Work out the finished part from the listing and answer in its coordinate system (mm). Face numbers are marked on the shaded views. A direction names the side the tool comes from. Coordinates: 2 decimals unless noted, no trailing zeros. Order: outer loops, then holes, each group sorted by start corner. A loop starts at its lowest first (then second) coordinate and runs counter-clockwise, first axis right, second up. Notation, with made-up numbers: M -27,51 L -11,51 A25 cw -11,84 Z; hole C 60.25,-28 d4. An arc over 180 degrees is marked long. Use a Markdown table: item, result.
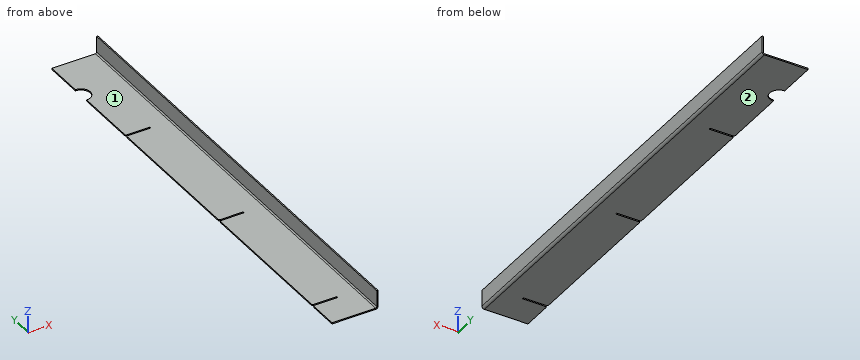
Autodesk Inventor part; units mm, degrees
ref_plane "YZ Plane" through (0, 0, 0) normal (1, 0, 0) x (0, 1, 0)
ref_plane "XZ Plane" through (0, 0, 0) normal (0, 1, 0) x (-1, 0, 0)
ref_plane "XY Plane" through (0, 0, 0) normal (0, 0, 1) x (1, 0, 0)
sketch "Sketch1" plane through (0, 0, 0) normal (0, 0, 1) x (1, 0, 0)
  line L0 (0, 0) -> (-144.8838, 0)
  line L1 (-144.8838, 0) -> (-144.8838, -1490)
  line L2 (-144.8838, -1490) -> (0, -1490)
  line L3 (0, -1490) -> (0, 0)
  line L4 (-144.8838, -1390) -> (-66, -1390)
  line L5 (-66, -1390) -> (-66, -1385)
  line L6 (-66, -1385) -> (-144.8838, -1385)
  line L7 (-144.8838, -1385) -> (-144.8838, -1390)
  line L8 (-144.8838, -893.3333) -> (-66, -893.3333)
  line L9 (-66, -893.3333) -> (-66, -888.3333)
  line L10 (-66, -888.3333) -> (-144.8838, -888.3333)
  line L11 (-144.8838, -888.3333) -> (-144.8838, -893.3333)
  line L12 (-144.8838, -396.6667) -> (-66, -396.6667)
  line L13 (-66, -396.6667) -> (-66, -391.6667)
  line L14 (-66, -391.6667) -> (-144.8838, -391.6667)
  line L15 (-144.8838, -391.6667) -> (-144.8838, -396.6667)
  circle A0 centre (-144.8838, -155) radius 30
  point P0 (-144.8838, -391.6667)
  point P1 (-144.8838, -1385)
  point P2 (-144.8838, -125)
  point P3 (-144.8838, -185)
  dimension "d0" = 1490
  dimension "d1" = 144.8838
  dimension "d2" = 5
  dimension "d4" = 100
  dimension "d7" = 496.6667
  dimension "d23" = 66
  dimension "d28" = 60
  dimension "d29" = 1335
extrude "Plate1" add sketch "Sketch1" along normal blind 4 contours L3 L2 L1 L4 L5 L6 L8 L9 L10 L12 L13 L14 A0 L0
sketch "Sketch2" plane through (4, 0, 0) normal (-1, 0, 0) x (0, -1, 0)
  line L0 (1490, 0) -> (0, 0)
  line L1 (0, 0) -> (0, 60)
  line L2 (0, 60) -> (1490, 60)
  line L3 (1490, 60) -> (1490, 0)
edge flange "Flange1" height 60 angle 90 thickness 4 bend radius 4 thickness toward (-1, 0, 0) relief tear relief width 4 relief depth 2 edges at (0, -745, 4) wall of the first edge with corners at (4, -1490, 0) (4, 0, 0) (4, 0, 60) (4, -1490, 60)
bend "Bend1"
corner "Corner1"
chamfer "Corner Chamfer1" distance 3 angle 45 6 edges at (-144.8838, -1390, 2) (-144.8838, -1385, 2) (-144.8838, -893.3333, 2) (-144.8838, -888.3333, 2) (-144.8838, -391.6667, 2) (-144.8838, -396.6667, 2)
equation "\"d0\" = Стрингер_длина"
equation "\"d1\" = стрингер_глубина_5"
equation "\"d2\" = паз_под_стрингер_толщина"
equation "\"d7\" = 0.333333 * Стрингер_длина"
equation "\"d23\" = паз_под_стрингер_глубина - Thickness"
equation "\"d28\" = 2 * радиус_выреза_под_сварку"
equation "\"d12\" = Thickness"
equation "\"d13\" = BendReliefWidth"
equation "\"d14\" = BendReliefDepth"
equation "\"d15\" = MinimumRemnant"
equation "\"d16\" = TransitionRadius"
equation "\"d17\" = ребро_усилителей"
equation "\"d19\" = BendRadius"
equation "\"d20\" = CornerReliefSize"
equation "\"d21\" = GapSize"
equation "\"d22\" = JacobiRadiusSize"
equation "\"BendRadius\" = Thickness"
equation "\"BendReliefWidth\" = Thickness"
equation "\"BendReliefDepth\" = 0.5 * Thickness"
equation "\"CornerReliefSize\" = 4 * Thickness"
equation "\"MinimumRemnant\" = 2 * Thickness"
equation "\"TransitionRadius\" = BendRadius"
equation "\"JacobiRadiusSize\" = BendRadius"
equation "\"GapSize\" = Thickness"
properties part number "GBK 0203 stringer 5" material "Steel"
1. Section C-C on x = -24.5 is taken. Determine the outline of the cut face in (y, z), then the cut area to 3 significant figures.
Answers below:
| item | result |
|---|---|
| outline | M -1490,0 L 0,0 L 0,4 L -1490,4 Z |
| area | 5,960 mm² |
2. Section D-D on z = 37.5 is taken. Determine the outline of the cut face in (x, y), then the cut area to 3 significant figures.
Answers below:
| item | result |
|---|---|
| outline | M 0,-1490 L 4,-1490 L 4,0 L 0,0 Z |
| area | 5,960 mm² |
3. Section A-A on x = -93 is taken. Determine the outline of the cut face in (y, z).
Answers below:
| item | result |
|---|---|
| outline | M -1490,0 L -1390,0 L -1390,4 L -1490,4 Z; M -1385,0 L -893.33,0 L -893.33,4 L -1385,4 Z; M -888.33,0 L -396.67,0 L -396.67,4 L -888.33,4 Z; M -391.67,0 L 0,0 L 0,4 L -391.67,4 Z |
4. Find the intervals of material crossed by probe 1 along Z at (x, y) = (-112, -484); probe 2 along Z at (x, y) = (-2, -321), in increasing order.
Answers below:
| item | result |
|---|---|
| probe 1 | 0 to 4 |
| probe 2 | 0.25 to 4.54 |
5. For the marked faces 1 and 2, determine the directions among +Z, -Z, +X, -X, +Y, -Y from which every point of the face is accessible in a straight line to the end or side of a thin tool.
Answers below:
| item | result |
|---|---|
| face 1 | +Z, -X, +Y, -Y |
| face 2 | -Z, +X, -X, +Y, -Y |
6. Section B-B on y = -616.5 is taken. Determine the outline of the cut face in (x, z), then the cut area to 3 significant figures.
Answers below:
| item | result |
|---|---|
| outline | M -144.88,0 L -4,0 A8 ccw 4,8 L 4,60 L 0,60 L 0,8 A4 cw -4,4 L -144.88,4 Z |
| area | 809 mm² |
7. Flat-ended cylindrical pins translate along their axes: P1, Ø1, axis at x = -25.5, y = -1224, coming from the +Z side; P2, Ø1, axis at y = -673.5, z = 17, coming from the -X side; P3, Ø2, axis at y = -395, z = 3, coming from the -X side. Find the tip coordinate at first contact, or state that the pin passes through.
Answers below:
| item | result |
|---|---|
| P1 | z = 4 |
| P2 | x = 0 |
| P3 | x = -66 |
